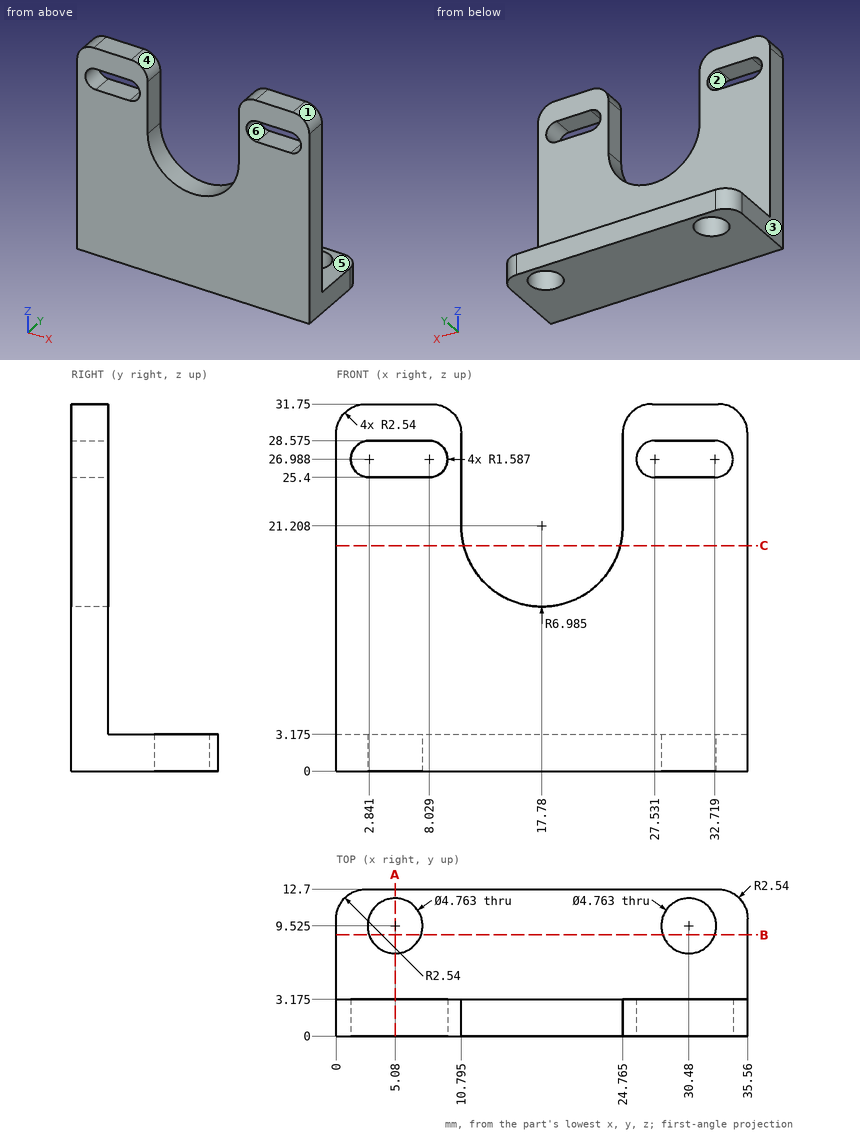
Job drawing, mm, ordinate dimensions from the low corner. One solid piece. A direction names the side the tool comes from. Round coordinates to 2 decimals unless told otherwise and drop trailing zeros. Order: outer loops, then holes, each group sorted by start corner. A loop starts at its lowest first (then second) coordinate and runs counter-clockwise, first axis right, second up. Notation, with made-up numbers: M -31,54 L -1,54 A20 cw -1,62 Z; hole C 57,65 d3. An arc over 180 degrees is marked long. Write each question's results on one line, items separated by ' | '. Start each with the question number.
(1) Saw through at A-A, the plane x = 5.08. State how many separate pieces and enclosed holes the cut face has, then the cut area to 3 significant figures.
(2) Saw through at C-C, the plane z = 19.5. Give the cut face in (x, y) (1 decimal).
(3) Drop flat-ended pins along their axis: pin 1 (8.5 mm diameter, centred on x = 26.5, z = 12, fed in from +Y) (1 decimal); pin 2 (3 mm diameter, centred on x = 23, y = 9.5, fed in from +Z) (1 decimal). Give the stop position or say it passes through.
(4) Saw through at B-B, the plane y = 8.75. Give the cut face in (x, z) (1 decimal).
(5) Probe probe 1 along X at (y, z) = (0.5, 22) (1 decimal); probe 2 along Y at (x, z) = (5.08, 2.1); probe 3 along Y at (x, z) = (13, 3.5) (1 decimal). List the from-to ranges inside material, lowest first. Write a range as from..to.
(6) Which spindle directions (+Z, -Z, +X, -X, +Y, -Y) get a long thin tool onto all of the face, cutting with end or side? Do the marked faces 4, 5 and 6. Say none if no direction does.
(7) Two-plate mould, pull along Z, no slides. Class the marked faces 1, 2 and 3: pulls with the +Z half, pulls with the -Z half, needs draft (parallel to the pull), parting line crosses it, or undercut.
Established:
1) separate pieces: 3 | enclosed holes: 0 | area: 106 mm^2
2) outline: M 0,0 L 11,0 L 11,3.2 L 0,3.2 Z; M 24.6,0 L 35.6,0 L 35.6,3.2 L 24.6,3.2 Z
3) pin 1: stops at y = 3.2 | pin 2: stops at z = 3.2
4) outline: M 0,0 L 2.8,0 L 2.8,3.2 L 0,3.2 Z; M 7.3,0 L 28.2,0 L 28.2,3.2 L 7.3,3.2 Z; M 32.7,0 L 35.6,0 L 35.6,3.2 L 32.7,3.2 Z
5) probe 1: x = 0..10.8, 24.8..35.6 | probe 2: y = 0..7.14, 11.91..12.7 | probe 3: y = 0..3.2
6) face 4: +Z, +Y, -Y | face 5: +Z, +X, -X, +Y | face 6: +Y, -Y
7) face 1: pulls with the +Z half | face 2: undercut | face 3: needs draft
